Geometry check sheet. Reference: the model listing, model coordinates, mm. A direction names the side the tool comes from. Coordinates: 2 decimals unless noted, no trailing zeros. Loops run counter-clockwise (first coordinate to the right, second up) from the corner with the lowest first, then second, coordinate; pieces in that order, holes last.
from build123d import *

# Parameters (mm, degrees)
BOSS_EXTRUDE1_DEPTH     = 5
CHAMFER1_SIZE           = 1
SKETCH2_R               = 1.8
CUT_EXTRUDE1_DEPTH      = 3
CUT_EXTRUDE1_DEPTH_BACK = 3
FILLET1_R               = 1.5
CHAMFER2_SIZE           = 1.5


with BuildPart() as part:
    # Sketch1 → Boss-Extrude1 (new body, symmetric)
    with BuildSketch(Plane(origin=(0, 0, 0), x_dir=(0, 0, -1), z_dir=(1, 0, 0))):
        Polygon((-5.25, -4.15), (-5.25, -6.15), (6.75, -6.15), (6.75, 6.15), (2.25, 6.15), (2.25, 4.15), (5.25, 4.15), (5.25, 1.85), (0.25, 1.85), (0.25, -0.15), (5.25, -0.15), (5.25, -4.15), align=None)
    extrude(amount=BOSS_EXTRUDE1_DEPTH, both=True)

    # Chamfer1
    chamfer1_edges = [part.edges().sort_by_distance(p)[0] for p in [
        (0, -4.15, -5.25),
        (0, -0.15, -5.25),
    ]]
    chamfer(chamfer1_edges, length=CHAMFER1_SIZE)

    # Sketch2 → Cut-Extrude1 (cut, two sides)
    with BuildSketch(Plane(origin=(0, -4.15, 0), x_dir=(1, 0, 0), z_dir=(0, 1, 0))) as cut_extrude1_sk:
        with Locations((0, -1.15)):
            Circle(SKETCH2_R)
    extrude(amount=CUT_EXTRUDE1_DEPTH, mode=Mode.SUBTRACT)
    extrude(cut_extrude1_sk.sketch, amount=-CUT_EXTRUDE1_DEPTH_BACK, mode=Mode.SUBTRACT)

    # Fillet1
    fillet1_edges = [part.edges().sort_by_distance(p)[0] for p in [
        (0, 6.15, -6.75),
        (0, -6.15, -6.75),
    ]]
    fillet(fillet1_edges, radius=FILLET1_R)

    # Chamfer2
    chamfer2_edges = [part.edges().sort_by_distance(p)[0] for p in [
        (0, 4.15, -2.25),
        (0, -0.15, -0.25),
    ]]
    chamfer(chamfer2_edges, length=CHAMFER2_SIZE)


solid = part.part
1) Section check D-D on z = 4.25. Record the cut outline in (x, y), and give its area (3 significant figures).
Data:
outline: (-5, -6.15) - (5, -6.15) - (5, -4.15) - (-5, -4.15) - close
area: 20.0 mm2
2) Mould release check, pull along Z, two halves, no side actions. Record for faces 3 (the flat face through (0, 1.85, -3)), 4 (the flat face through (0, 0, -6.75)), 5 (the cylindrical face through (1.717, -5.136, 0.609)): +Z half, -Z half, draft (parallel to the pull), parting line (faces both ways), or undercut.
Data:
face 3: draft
face 4: -Z half
face 5: undercut
3) Access from +Z, -Z, +X, -X, +Y, -Y to the whole of each face (thin tool, end or side, straight path). Record for faces 1 (the cylindrical face through (0.07, -5.72, -6.3)), 2 (the flat face through (-0.1, 4.9, -3)).
Data:
face 1: -Z, +X, -X, -Y
face 2: +Z, +X, -X
4) Depth check by flat-ended pin: pin 1 (1 mm diameter, centred on y = -3, z = -0.5, fed in from -X); pin 2 (2 mm diameter, centred on x = 3, z = 0, fed in from +Y); pin 3 (1.6 mm diameter, centred on x = -0.5, y = -2, fed in from +Z); pin 4 (2.5 mm diameter, centred on x = 2, y = 3, fed in from +Z). Enter the tip coordinate at first touch or a pass-through.
Data:
pin 1: passes through
pin 2: stops at y = 1.85
pin 3: stops at z = -5.25
pin 4: stops at z = -0.25
5) Section check B-B on z = 1.15. Record the cut outline in (x, y), and give its area (3 significant figures).
Data:
outline: (-5, -6.15) - (-1.8, -6.15) - (-1.8, -4.15) - (-5, -4.15) - close; (1.8, -6.15) - (5, -6.15) - (5, -4.15) - (1.8, -4.15) - close
area: 12.8 mm2
6) Material ranges on probe 1 along Y at (x, z) = (-0.5, -4); probe 2 along Y at (x, z) = (1.75, -3.25); probe 3 along X at (y, z) = (-4.65, 1.15), recorded low to high.
Data:
probe 1: y = -6.15 to -4.15, -0.15 to 1.85, 4.15 to 6.15
probe 2: y = -6.15 to -4.15, -0.15 to 1.85, 4.65 to 6.15
probe 3: x = -5 to -1.8, 1.8 to 5
7) Section check C-C on x = 2. Record the cut outline in (y, z), and give its area (3 significant figures).
Data:
outline: (-6.15, -5.25) arc R1.5 ccw to (-4.65, -6.75) - (4.65, -6.75) arc R1.5 ccw to (6.15, -5.25) - (6.15, -2.25) - (5.65, -2.25) - (4.15, -3.75) - (4.15, -5.25) - (1.85, -5.25) - (1.85, -0.25) - (1.35, -0.25) - (-0.15, -1.75) - (-0.15, -4.25) - (-1.15, -5.25) - (-3.15, -5.25) - (-4.15, -4.25) - (-4.15, 5.25) - (-6.15, 5.25) - close
area: 53.2 mm2
8) Section check A-A on x = 0. Record the cut outline in (y, z), and give its area (3 significant figures).
Data:
outline: (-6.15, -5.25) arc R1.5 ccw to (-4.65, -6.75) - (4.65, -6.75) arc R1.5 ccw to (6.15, -5.25) - (6.15, -2.25) - (5.65, -2.25) - (4.15, -3.75) - (4.15, -5.25) - (1.85, -5.25) - (1.85, -0.25) - (1.35, -0.25) - (-0.15, -1.75) - (-0.15, -4.25) - (-1.15, -5.25) - (-3.15, -5.25) - (-4.15, -4.25) - (-4.15, -0.65) - (-6.15, -0.65) - close; (-6.15, 2.95) - (-4.15, 2.95) - (-4.15, 5.25) - (-6.15, 5.25) - close
area: 46.0 mm2
